from build123d import *

# Parameters (mm, degrees)
SKETCH1_W           = 51
SKETCH1_H           = 22.8
BOSS_EXTRUDE1_DEPTH = 3
SKETCH2_W           = 4
SKETCH2_H           = 5
BOSS_EXTRUDE2_DEPTH = 2.5
SKETCH3_W           = 7
SKETCH3_H           = 7
BOSS_EXTRUDE3_DEPTH = 5
SKETCH4_R           = 1.27
CUT_EXTRUDE1_DEPTH  = 57.087788332
FILLET1_R           = 3
SKETCH5_R           = 0.75
CUT_EXTRUDE2_DEPTH  = 57.087788332


with BuildPart() as part:
    # Sketch1 → Boss-Extrude1 (new body)
    with BuildSketch(Plane(origin=(0, 0, 0), x_dir=(1, 0, 0), z_dir=(0, 1, 0))):
        with Locations((25.5, 11.4)):
            Rectangle(SKETCH1_W, SKETCH1_H)
    extrude(amount=BOSS_EXTRUDE1_DEPTH)

    # Sketch2 → Boss-Extrude2 (add)
    with BuildSketch(Plane(origin=(0, 3, 0), x_dir=(1, 0, 0), z_dir=(0, 1, 0))):
        with Locations((2, 11.4)):
            Rectangle(SKETCH2_W, SKETCH2_H)
    extrude(amount=BOSS_EXTRUDE2_DEPTH)

    # Sketch3 → Boss-Extrude3 (add)
    with BuildSketch(Plane(origin=(0, 3, 0), x_dir=(1, 0, 0), z_dir=(0, 1, 0))):
        with Locations((10.5, 19.3)):
            Rectangle(SKETCH3_W, SKETCH3_H)
    extrude(amount=BOSS_EXTRUDE3_DEPTH)

    # Sketch4 → Cut-Extrude1 (cut, through all)
    with BuildSketch(Plane(origin=(0, 3, 0), x_dir=(1, 0, 0), z_dir=(0, 1, 0))):
        with Locations(Location((2.54, 20.26, 0), (0, 0, 270))):
            Circle(SKETCH4_R)
        with Locations(Location((2.54, 2.54, 0), (0, 0, 270))):
            Circle(SKETCH4_R)
        with Locations(Location((48.46, 20.26, 0), (0, 0, 270))):
            Circle(SKETCH4_R)
        with Locations(Location((48.46, 2.54, 0), (0, 0, 270))):
            Circle(SKETCH4_R)
    extrude(amount=-CUT_EXTRUDE1_DEPTH, mode=Mode.SUBTRACT)

    # Fillet1
    fillet1_edges = [part.edges().sort_by_distance(p)[0] for p in [
        (0, 1.5, 0),
        (0, 1.5, -22.8),
        (51, 1.5, -22.8),
        (51, 1.5, 0),
    ]]
    fillet(fillet1_edges, radius=FILLET1_R)

    # Sketch5 → Cut-Extrude2 (cut, through all)
    with BuildSketch(Plane(origin=(0, 3, 0), x_dir=(1, 0, 0), z_dir=(0, 1, 0))):
        with Locations(Location((47.27309584, 6.32, 0), (0, 0, 270))):
            Circle(SKETCH5_R)
        with Locations(Location((49.81309584, 8.86, 0), (0, 0, 270))):
            Circle(SKETCH5_R)
        with Locations(Location((44.73309584, 16.48, 0), (0, 0, 270))):
            Circle(SKETCH5_R)
        with Locations(Location((39.65309584, 6.32, 0), (0, 0, 270))):
            Circle(SKETCH5_R)
        with Locations(Location((42.19309584, 6.32, 0), (0, 0, 270))):
            Circle(SKETCH5_R)
        with Locations(Location((44.73309584, 6.32, 0), (0, 0, 270))):
            Circle(SKETCH5_R)
        with Locations(Location((49.81309584, 6.32, 0), (0, 0, 270))):
            Circle(SKETCH5_R)
        with Locations(Location((47.27309584, 8.86, 0), (0, 0, 270))):
            Circle(SKETCH5_R)
        with Locations(Location((44.73309584, 8.86, 0), (0, 0, 270))):
            Circle(SKETCH5_R)
        with Locations(Location((42.19309584, 8.86, 0), (0, 0, 270))):
            Circle(SKETCH5_R)
        with Locations(Location((39.65309584, 8.86, 0), (0, 0, 270))):
            Circle(SKETCH5_R)
        with Locations(Location((39.65309584, 11.4, 0), (0, 0, 270))):
            Circle(SKETCH5_R)
        with Locations(Location((42.19309584, 11.4, 0), (0, 0, 270))):
            Circle(SKETCH5_R)
        with Locations(Location((44.73309584, 11.4, 0), (0, 0, 270))):
            Circle(SKETCH5_R)
        with Locations(Location((47.27309584, 11.4, 0), (0, 0, 270))):
            Circle(SKETCH5_R)
        with Locations(Location((49.81309584, 11.4, 0), (0, 0, 270))):
            Circle(SKETCH5_R)
        with Locations(Location((49.81309584, 13.94, 0), (0, 0, 270))):
            Circle(SKETCH5_R)
        with Locations(Location((47.27309584, 13.94, 0), (0, 0, 270))):
            Circle(SKETCH5_R)
        with Locations(Location((44.73309584, 13.94, 0), (0, 0, 270))):
            Circle(SKETCH5_R)
        with Locations(Location((42.19309584, 13.94, 0), (0, 0, 270))):
            Circle(SKETCH5_R)
        with Locations(Location((39.65309584, 13.94, 0), (0, 0, 270))):
            Circle(SKETCH5_R)
        with Locations(Location((39.65309584, 16.48, 0), (0, 0, 270))):
            Circle(SKETCH5_R)
        with Locations(Location((42.19309584, 16.48, 0), (0, 0, 270))):
            Circle(SKETCH5_R)
        with Locations(Location((47.27309584, 16.48, 0), (0, 0, 270))):
            Circle(SKETCH5_R)
        with Locations(Location((49.81309584, 16.48, 0), (0, 0, 270))):
            Circle(SKETCH5_R)
    extrude(amount=-CUT_EXTRUDE2_DEPTH, mode=Mode.SUBTRACT)


solid = part.part
Model file for the job. Use its own axes, mm. A direction names the side the tool comes from. Give positions to 0.01 mm unless a question says otherwise; leave off trailing zeros. Write each loop counter-clockwise with the first axis right and the second up, starting at its lowest first coordinate (ties: lowest second). Pieces come first, ordered by that corner, then holes. Notation, with made-up numbers: M 50,-23.5 L 78,-23.5 A25 cw 78,0.5 Z; hole C 71.25,4.25 d4. An arc over 180 degrees is marked long. One line per item, written item: value. Start each with the question number.
Q1. Saw through at D-D, the plane x = 2.54. Write the cut outline in (y, z).
Q2. Saw through at A-A, the plane z = -6.32. Write the cut outline in (x, y), plus the area to 4 significant figures.
Q3. Saw through at B-B, the plane y = 4. Write the cut outline in (x, z).
Q4. Drop flat-ended pins along their axis: pin 1 Ø1.7 at (x, z) = (47.27, -16.48) entering from -Y; pin 2 Ø2.5 at (y, z) = (4.5, -17.5) entering from -X; pin 3 Ø4.5 at (x, z) = (2, -11.5) entering from +Y; pin 4 Ø2.5 at (x, z) = (49.81, -6.32) entering from +Y. Give the stop position or say it passes through.
Q5. Saw through at C-C, the plane z = -20.26. Write the cut outline in (x, y), plus the area to 3 significant figures.
Q6. Two-plate mould, pull along X, no slides. Class faces 4 (the flat face through (25, 0, -12)), 5 (the cylindrical face through (50.1, 1.52, -0.86)), 6 (the cylindrical face through (45.365, 1.521, -8.457)): +X half, -X half, draft (parallel to the pull), parting line (faces both ways), or undercut.
Q7. Probe probe 1 along X at (y, z) = (1.05, -8.86); probe 2 along X at (y, z) = (2.05, -20.26); probe 3 along X at (y, z) = (1.25, -12). List the from-to ranges inside material, lowest first. Write a range as [from, to].
Q8. 3-axis set-ups, long thin cutter, end or side, ignore diameter. For faces 1 (the flat face through (14, 5, -19)), 2 (the flat face through (10, 5, -15.8)), 3 (the cylindrical face through (42.8, 1.5, -13.5)): which of +Z, -Z, +X, -X, +Y, -Y reach the whole face in a straight line?
Output values:
1. outline: M 0,-22.76 L 3,-22.76 L 3,-21.53 L 0,-21.53 Z; M 0,-18.99 L 3,-18.99 L 3,-13.9 L 5.5,-13.9 L 5.5,-8.9 L 3,-8.9 L 3,-3.81 L 0,-3.81 Z; M 0,-1.27 L 3,-1.27 L 3,-0.04 L 0,-0.04 Z
2. outline: M 0,0 L 38.9,0 L 38.9,3 L 0,3 Z; M 40.4,0 L 41.44,0 L 41.44,3 L 40.4,3 Z; M 42.94,0 L 43.98,0 L 43.98,3 L 42.94,3 Z; M 45.48,0 L 46.52,0 L 46.52,3 L 45.48,3 Z; M 48.02,0 L 49.06,0 L 49.06,3 L 48.02,3 Z; M 50.56,0 L 51,0 L 51,3 L 50.56,3 Z
2. area: 130.5 mm²
3. outline: M 0,-13.9 L 4,-13.9 L 4,-8.9 L 0,-8.9 Z; M 7,-22.8 L 14,-22.8 L 14,-15.8 L 7,-15.8 Z
4. pin 1: stops at y = 0
4. pin 2: stops at x = 7
4. pin 3: stops at y = 5.5
4. pin 4: stops at y = 3
5. outline: M 0.04,0 L 1.27,0 L 1.27,3 L 0.04,3 Z; M 3.81,0 L 47.19,0 L 47.19,3 L 14,3 L 14,8 L 7,8 L 7,3 L 3.81,3 Z; M 49.73,0 L 50.96,0 L 50.96,3 L 49.73,3 Z
5. area: 173 mm²
6. face 4: draft
6. face 5: +X half
6. face 6: undercut
7. probe 1: x = [0, 38.9], [40.4, 41.44], [42.94, 43.98], [45.48, 46.52], [48.02, 49.06], [50.56, 51]
7. probe 2: x = [0.04, 1.27], [3.81, 47.19], [49.73, 50.96]
7. probe 3: x = [0, 39.2], [40.1, 41.74], [42.64, 44.28], [45.18, 46.82], [47.72, 49.36], [50.26, 51]
8. face 1: +Z, -Z, +X, +Y
8. face 2: +Z, +X, -X, +Y
8. face 3: +Y, -Y
